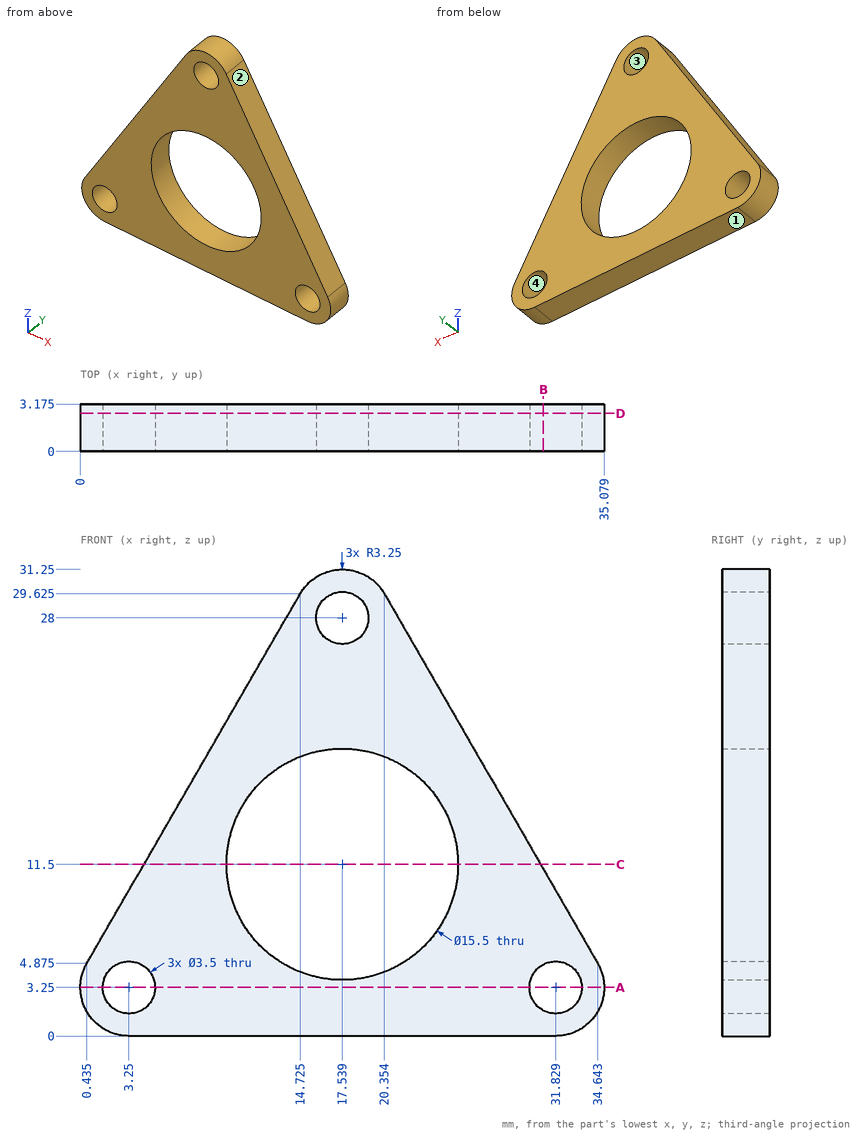
For this review, use the dimensioned drawing (mm, ordinates from the lowest corner) and the shaded views. Round coordinates to 2 decimals unless told otherwise and drop trailing zeros. Loops run counter-clockwise (first coordinate to the right, second up) from the corner with the lowest first, then second, coordinate; pieces in that order, holes last. Notation, with made-up numbers: (15.5, 48.5) -> (50.5, 48.5) arc R29 cw to (50.5, 78.5) -> close; hole circle Ø7 at (83.25, 68.5). An arc over 180 degrees is marked (long way). Write item = value, one per line. Start each with the question number.
Item 1: Take a section at D-D on y = 2.55. Count the separate pieces of the cut face and the enclosed holes in it, plus the area to 3 significant figures.
Item 2: Mouldability with a two-part tool opening along X and no side actions: class the marked faces 1, 2, 3 and 4 as released by +X, released by -X, zero draft, split by the parting line, or undercut.
Item 3: Take a section at B-B on x = 31. Give the boundary of the cut face in (y, z) (1 decimal).
Item 4: To check wall thickness, follow L1, parallel to X at y = 1.1, z = 3.25; L2, parallel to X at y = 2.45, z = 2.5; L3, parallel to Z at x = 31, y = 0.75 (1 decimal). State the ranges of each line that lie inside material, in increasing order.
Item 5: Take a section at C-C on z = 11.5. Give the boundary of the cut face in (x, y) (1 decimal).
Item 6: Take a section at A-A on z = 3.25. Give the boundary of the cut face in (x, y) (1 decimal).
Item 7: Insertion check: pin 1 (1.5 mm diameter, centred on x = 9.5, z = 20, fed in from -Y); pin 2 (1 mm diameter, centred on y = 0.5, z = 6.5, fed in from -X) (1 decimal). Each pin has a flat end and moves straight along its axis. Give the tip position at first contact, or say it passes through.
Result:
q1.separate_pieces = 1
q1.enclosed_holes = 4
q1.area = 448 mm²
q2.face_1 = zero draft
q2.face_2 = released by +X
q2.face_3 = undercut
q2.face_4 = undercut
q3.outline = (0, 0) -> (3.2, 0) -> (3.2, 1.7) -> (0, 1.7) -> close; (0, 4.8) -> (3.2, 4.8) -> (3.2, 11.2) -> (0, 11.2) -> close
q4.L1 = 0 to 1.5, 5 to 30.08, 33.58 to 35.08
q4.L2 = 0.09 to 1.67, 4.83 to 30.25, 33.41 to 34.99
q4.L3 = 0 to 1.7, 4.8 to 11.2
q5.outline = (4.3, 0) -> (9.8, 0) -> (9.8, 3.2) -> (4.3, 3.2) -> close; (25.3, 0) -> (30.8, 0) -> (30.8, 3.2) -> (25.3, 3.2) -> close
q6.outline = (0, 0) -> (1.5, 0) -> (1.5, 3.2) -> (0, 3.2) -> close; (5, 0) -> (30.1, 0) -> (30.1, 3.2) -> (5, 3.2) -> close; (33.6, 0) -> (35.1, 0) -> (35.1, 3.2) -> (33.6, 3.2) -> close
q7.pin_1 = 0
q7.pin_2 = 1.1
